The model under review builds one solid part; all positions refer to its coordinate system, in mm. Round coordinates to 2 decimals unless told otherwise and drop trailing zeros. Write each loop counter-clockwise with the first axis right and the second up, starting at its lowest first coordinate (ties: lowest second). Pieces come first, ordered by that corner, then holes.
Item 1: Clearance check with flat-ended pins moving along their axes: pin 1 Ø2.5 at (x, y) = (21.89, -17.45) entering from -Z; pin 2 Ø5 at (x, y) = (-27.3, 6.23) entering from -Z; pin 3 Ø1.5 at (y, z) = (20.5, 0.5) entering from -X; pin 4 Ø1.5 at (x, z) = (-23, 0.5) entering from -Y. State where each tip first meets the part, or that it passes through.
Item 2: To check wall thickness, follow L1, parallel to Y at x = -11, z = 0.75; L2, parallel to Y at x = 20.5, z = 1.95; L3, parallel to Y at x = -16, z = 1.15. State the ranges of each line that lie inside material, in increasing order.
Item 3: Add section B-B (x = 5.5). Give the boundary of the cut face in (y, z), plus the area to 3 significant figures.
Item 4: Add section C-C (z = 2.4). Give the boundary of the cut face in (x, y) (1 decimal).
Item 5: Add section A-A (y = -22.5). Give the boundary of the cut face in (x, z).
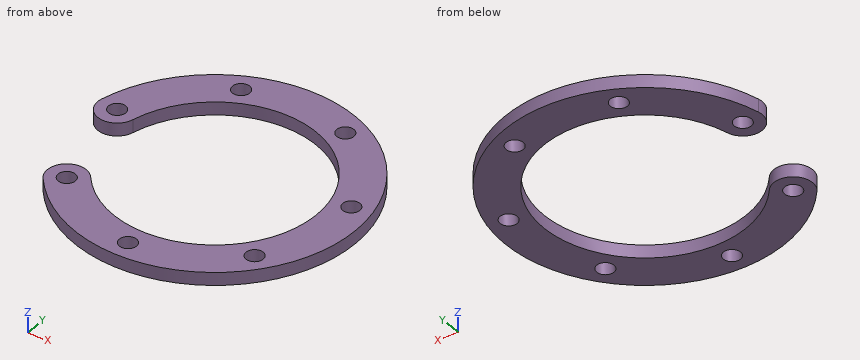
Autodesk Inventor part; units mm, degrees
ref_plane "YZ Plane" through (0, 0, 0) normal (1, 0, 0) x (0, 1, 0)
ref_plane "XZ Plane" through (0, 0, 0) normal (0, 1, 0) x (-1, 0, 0)
ref_plane "XY Plane" through (0, 0, 0) normal (0, 0, 1) x (1, 0, 0)
sketch "Sketch1" plane through (0, 0, 0) normal (0, 0, 1) x (1, 0, 0)
  arc A0 (-25.407, -20.2666) -> (-31.6861, 7.228) centre (0, 0) ccw
  arc A1 (-18.3712, -14.6543) -> (-22.9115, 5.2264) centre (0, 0) ccw
  circle A2 centre (27.2972, 6.234) radius 2
  circle A3 centre (12.1456, 25.2286) radius 2
  circle A4 centre (-12.1519, 25.2256) radius 2
  circle A5 centre (-27.2988, 6.2272) radius 2
  circle A6 centre (-21.8891, -17.4604) radius 2
  circle A7 centre (0.0035, -28) radius 2
  circle A8 centre (21.8935, -17.455) radius 2
  arc A9 (-18.3712, -14.6543) -> (-25.407, -20.2666) centre (-21.8891, -17.4604) ccw
  arc A10 (-31.6861, 7.228) -> (-22.9115, 5.2264) centre (-27.2988, 6.2272) ccw
  line L0 (0, 0) -> (-27.2988, 6.2272)
  line L1 (0, 0) -> (-28.0096, 0)
  dimension "d0" = 65
  dimension "d1" = 47
  dimension "d2" = 4
  dimension "d5" = 360
  dimension "d7" = 9
  dimension "d8" = 9
  dimension "d11" = 12.85
  dimension "d12" = 54.596
extrude "Extrusion1" add sketch "Sketch1" along normal blind 3
properties part number "fin entraineur"
Numbers:
1. pin 1: passes through
1. pin 2: stops at z = 0
1. pin 3: stops at x = -25.81
1. pin 4: stops at y = -23.69
2. L1: y = -30.58 to -20.77, 20.77 to 23.59, 26.86 to 30.58
2. L2: y = -25.22 to -18.89, -16.02 to -11.49, 11.49 to 25.22
2. L3: y = -28.29 to -17.21, 17.21 to 28.29
3. outline: (-32.03, 0) - (-22.85, 0) - (-22.85, 3) - (-32.03, 3) - close; (22.85, 0) - (32.03, 0) - (32.03, 3) - (22.85, 3) - close
3. area: 55.1 mm2
4. outline: (-31.7, 7.2) arc R4.5 ccw to (-22.9, 5.2) arc R23.5 cw (long way) to (-18.4, -14.7) arc R4.5 ccw to (-25.4, -20.3) arc R32.5 ccw (long way) to start; hole circle Ø4 at (-27.3, 6.2); hole circle Ø4 at (-21.9, -17.5); hole circle Ø4 at (-12.2, 25.2); hole circle Ø4 at (0, -28); hole circle Ø4 at (12.1, 25.2); hole circle Ø4 at (21.9, -17.5); hole circle Ø4 at (27.3, 6.2)
5. outline: (-23.45, 0) - (-6.78, 0) - (-6.78, 3) - (-23.45, 3) - close; (6.78, 0) - (23.45, 0) - (23.45, 3) - (6.78, 3) - close
